For this review, take the finished solid that the model builds, in its own axes (mm). A direction names the side the tool comes from. Coordinates: 2 decimals unless noted, no trailing zeros. Loops run counter-clockwise (first coordinate to the right, second up) from the corner with the lowest first, then second, coordinate; pieces in that order, holes last. Notation, with made-up numbers: (70.5, 73.5) - (111.5, 73.5) arc R31 cw to (111.5, 102.5) - close; hole circle Ø4 at (-11.75, 49.25). An arc over 180 degrees is marked (long way). One line per item, written item: value. Start each with the question number.
1. For faces 1 (the face through (20, -49, 140)), 2 (the face through (100, -80, 10)), 3 (the face through (90, -50, 9)), list the 3-axis set-ups (+Z, -Z, +X, -X, +Y, -Y) from which the entire face can be reached by the end or side of a thin tool; tool diameter is ignored.
2. To check wall thickness, follow line 1 (Y direction, x = 82, z = 64); line 2 (Z direction, x = 33, y = -9); line 3 (X direction, y = -93, z = 143). State the ranges of each line that lie inside material, in increasing order. Write a range as from..to.
3. Take a section at B-B, the plane z = 82. State the section outline as (x, y) points, and give its area (3 significant figures).
4. Insertion check: pin 1 (3 mm diameter, centred on y = -24, z = 117, fed in from +X); pin 2 (6 mm diameter, centred on x = 34.5, y = -70.5, fed in from +Z); pin 3 (2 mm diameter, centred on x = 20.5, y = -40, fed in from +Z); pin 4 (6 mm diameter, centred on y = -27, z = 144.5, fed in from +X). Each pin has a flat end and moves straight along its axis. Give the tip position at first contact, or say it passes through.
5. Take a section at D-D, the plane x = 57.5. State the section outline as (y, z) points.
6. The part is to be moulded in two halves that separate along Z. For faces 4 (the face through (69.97, -50.14, 83.68)), 5 (the face through (55.338, -50.14, 148.552)), 6 (the face through (49, -49, 0)), 7 (the face through (100, -20, 10)), say which applies: released by +Z, released by -Z, zero draft, split by the parting line, or undercut.
7. Take a section at C-C, the plane x = 78. State the section outline as (y, z) points.
8. Take a section at A-A, the plane y = -11. State the section outline as (x, z) points, and give its area (3 significant figures).
```python
from build123d import *

# Parameters (mm, degrees)
F1_DEPTH = 100
F3_W     = 20
F3_H     = 20
F4_DEPTH = 10
F2_W     = 20
F2_H     = 136
F5_DEPTH = 10
F6_DEPTH = 10
F7_W     = 20
F7_H     = 136
F8_DEPTH = 10


with BuildPart() as f1:
    # F0 (on Front) → F1 (new body)
    with BuildSketch(Plane.XZ):
        Polygon((0, 150), (0, 0), (100, 0), (100, 20), (60.0500312891, 150), (40, 150), (40, 130), (20, 130), (20, 150), align=None)
    extrude(amount=F1_DEPTH)

    # F3 (on face) → F4 (cut)
    with BuildSketch(Plane.YZ.offset(100)):
        with Locations((-50, 10)):
            Rectangle(F3_W, F3_H)
    extrude(amount=-F4_DEPTH, mode=Mode.SUBTRACT)

    # F2 (on face) → F5 (join)
    with BuildSketch(Plane(origin=(96.9869116916, 0, 29.8048006727), x_dir=(0, 1, 0), z_dir=(0.9558823529, 0, 0.2937497699))):
        with Locations((-50, 57.7426700655)):
            Rectangle(F2_W, F2_H)
    extrude(amount=F5_DEPTH)

    # F6 (cut): a face of the model
    f6_faces = [f1.faces().sort_by_distance(p)[0] for p in [
        (89.583839174, -50, 87.9374976993),
    ]]
    extrude(f6_faces, amount=-F6_DEPTH, mode=Mode.SUBTRACT)

    # F7 (on face) → F8 (cut)
    with BuildSketch(Plane(origin=(96.9869116916, 0, 29.8048006727), x_dir=(0, 1, 0), z_dir=(0.9558823529, 0, 0.2937497699))):
        with Locations((-50, 57.7426700655)):
            Rectangle(F7_W, F7_H)
    extrude(amount=-F8_DEPTH, mode=Mode.SUBTRACT)


solid = f1.part
```
Solutions:
1. face 1: +Z, +Y, -Y
1. face 2: +Z, -Z, +X, +Y, -Y
1. face 3: +Z, -Z, +X
2. line 1: -100..-60, -40..0
2. line 2: 0..130
2. line 3: 0..20, 40..62.2
3. outline: (0, -100) - (80.95, -100) - (80.95, -60) - (70.49, -60) - (70.49, -40) - (80.95, -40) - (80.95, 0) - (0, 0) - close
3. area: 7,890 mm2
4. pin 1: x = 70.65
4. pin 2: z = 130
4. pin 3: z = 150
4. pin 4: x = 62.66
5. outline: (-100, 0) - (0, 0) - (0, 150) - (-100, 150) - close; hole (-60, 124.26) - (-40, 124.26) - (-40, 149.22) - (-60, 149.22) - close
6. face 4: undercut
6. face 5: undercut
6. face 6: released by -Z
6. face 7: zero draft
7. outline: (-100, 0) - (0, 0) - (0, 91.59) - (-40, 91.59) - (-40, 57.55) - (-60, 57.55) - (-60, 91.59) - (-100, 91.59) - close
8. outline: (0, 0) - (100, 0) - (100, 20) - (60.05, 150) - (40, 150) - (40, 130) - (20, 130) - (20, 150) - (0, 150) - close
8. area: 12,000 mm2
